Can you work these out from the model? Positions are in its coordinate system, mm. Face numbers are marked on the shaded views. A direction names the side the tool comes from. Give positions to 0.01 mm unless a question says otherwise; leave off trailing zeros. Write each loop counter-clockwise with the first axis right and the second up, starting at its lowest first coordinate (ties: lowest second). Pieces come first, ordered by that corner, then holes.
1. Suppose I cut it at A-A (z = 0). Please give me the cut outline in (x, y), and give its area (3 significant figures).
2. I'm going to push a flat-ended pin straight in: pin 1 (1.5 mm diameter, centred on x = -10, y = -51.5, fed in from +Z). Where does the tip first touch, or does it pass through?
3. On a 3-axis mill with a long thin cutter (end or side, diameter ignored), from which of +Z, -Z, +X, -X, +Y, -Y can I reach the whole of each face in a straight line? I mean the marked faces 1 and 2. Say none if no direction works.
4. If I drill on probe 1 along Y at (x, z) = (-10.9, -1.25); probe 2 along Y at (x, z) = (-10.55, -0.5); probe 3 along Z at (x, y) = (-10.9, -47), over which ranges is the centre line in solid material (lowest first)?
5. Suppose I cut it at B-B (y = -50.5). Please give me the cut outline in (x, z), and give its area (3 significant figures).
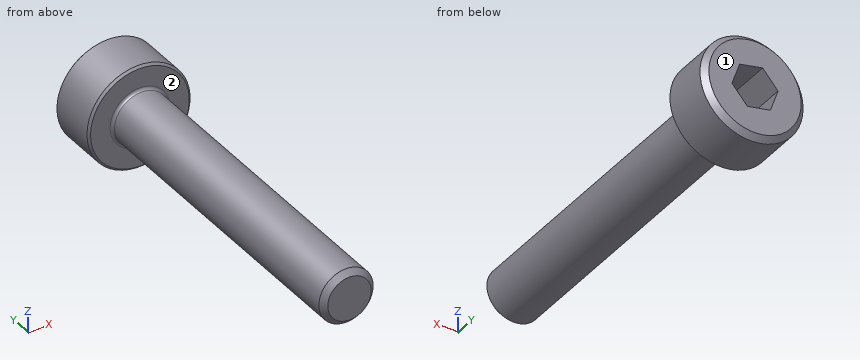
Autodesk Inventor part; units mm, degrees
ref_plane "YZ Plane" through (0, 0, 0) normal (1, 0, 0) x (0, 1, 0)
ref_plane "XZ Plane" through (0, 0, 0) normal (0, 1, 0) x (-1, 0, 0)
ref_plane "XY Plane" through (0, 0, 0) normal (0, 0, 1) x (1, 0, 0)
sketch "Sketch1" plane through (0, 0, 0) normal (0, 0, 1) x (1, 0, 0)
  line L0 (-10.9228, -43) -> (-12.8228, -43)
  line L1 (-12.8228, -43) -> (-12.8228, -41)
  line L2 (-12.8228, -41) -> (-10.9228, -41)
  line L3 (-10.9228, -41) -> (-10.9228, -43)
  line L4 (-10.9228, -43) -> (-10.9228, -55)
  line L5 (-10.9228, -55) -> (-11.9228, -55)
  line L6 (-11.9228, -55) -> (-11.9228, -43)
  dimension "d0" = 1.9
  dimension "d1" = 2
  dimension "d3" = 1
  dimension "d16" = 12
revolve "Revolution1" add sketch "Sketch1" angle 360 about axis through (-10.9228, -43, 0) along (0, -1, 0)
chamfer "Chamfer1" distance 0.2 angle 45 1 edges at (-9.0228, -41, 0)
sketch "Boceto2" plane through (-10.9228, -41, 0) normal (0, 1, 0) x (1, 0, 0)
  line L0 (0.5669, -0.6547) -> (-0.2835, -0.8183)
  line L1 (-0.2835, -0.8183) -> (-0.8504, -0.1636)
  line L2 (-0.8504, -0.1636) -> (-0.5669, 0.6547)
  line L3 (-0.5669, 0.6547) -> (0.2835, 0.8183)
  line L4 (0.2835, 0.8183) -> (0.8504, 0.1636)
  line L5 (0.8504, 0.1636) -> (0.5669, -0.6547)
  point P0 (10.9228, 0)
  point P1 (0, 0)
  dimension "d11" = 1.5
extrude "Extrusión1" cut sketch "Boceto2" against normal blind 2
fillet "Fillet1" radius 0.1 1 edges at (-9.9228, -43, 0)
chamfer "Chamfer3" distance 0.2 angle 45 1 edges at (-9.9228, -55, 0)
thread "Thread2"
chamfer "Chamfer4" distance 0.08 angle 45 1 edges at (-9.0228, -43, 0)
properties part number "Tornillo Allen cabeza cilindrica M2x16mm"
Checks:
1. outline: (-12.82, -42.92) - (-12.74, -43) - (-12.02, -43) arc R0.1 cw to (-11.92, -43.1) - (-11.92, -54.8) - (-11.72, -55) - (-10.12, -55) - (-9.92, -54.8) - (-9.92, -43.1) arc R0.1 cw to (-9.82, -43) - (-9.1, -43) - (-9.02, -42.92) - (-9.02, -41.2) - (-9.22, -41) - (-10.13, -41) - (-10.13, -43) - (-11.72, -43) - (-11.72, -41) - (-12.62, -41) - (-12.82, -41.2) - close
1. area: 28.3 mm2
2. pin 1: stops at z = 0.98
3. face 1: +Z, -Z, +X, -X, +Y
3. face 2: -Y
4. probe 1: y = -43 to -41
4. probe 2: y = -55 to -43
4. probe 3: z = -1 to 1
5. outline: circle Ø2 at (-10.92, 0)
5. area: 3.14 mm2
